from build123d import *

# Parameters (mm, degrees)
F0_R     = 1.905
F1_DEPTH = 5.08
F0_R_2   = 58.9915
F2_DEPTH = 10.16
F3_R     = 1.8415
F7_D     = 3.81
F7_DEPTH = 3.81
F7_TIP   = 1.1446394792


with BuildPart() as f1:
    # F0 (on Top) → F1 (new body)
    with BuildSketch(Plane.XY):
        Polygon((-6.4052528628, -3.7129219378), (-0.0261097385, -7.3959219378), (6.3530333858, -3.7129219378), (6.3530333858, 3.6530780622), (-0.0261097385, 7.3360780622), (-6.4052528628, 3.6530780622), align=None)
        with Locations((-0.0261097385, -0.0299219378)):
            Circle(F0_R, mode=Mode.SUBTRACT)
    extrude(amount=F1_DEPTH)

    # F0 (on Top) → F2 (join)
    with BuildSketch(Plane.XY):
        Circle(F0_R_2)
        with BuildLine():
            Line((-44.2124819173, 9.2097946363), (-23.9423226363, 4.6011586921))
            ThreePointArc((-23.9423226363, 4.6011586921), (-20.5137110236, 2.5239744907), (-19.0126005957, -1.1931129822))
            ThreePointArc((-19.0126005957, -1.1931129822), (-18.1042521178, -5.9277782732), (-16.0364137318, -10.2827979958))
            ThreePointArc((-16.0364137318, -10.2827979958), (-15.0448681501, -14.1162516757), (-16.5173341467, -17.7918976931))
            Line((-16.5173341467, -17.7918976931), (-29.9142206112, -33.7590248091))
            ThreePointArc((-29.9142206112, -33.7590248091), (-34.752324822, -36.0274693708), (-39.6091563625, -33.7994028387))
            ThreePointArc((-39.6091563625, -33.7994028387), (-49.423694035, -16.3885132924), (-51.9564452709, 3.4369601117))
            ThreePointArc((-51.9564452709, 3.4369601117), (-49.4154929179, 8.1088853878), (-44.2124819173, 9.2097946363))
        make_face(mode=Mode.SUBTRACT)
        Polygon((6.3530333858, -3.7129219378), (-0.0261097385, -7.3959219378), (-6.4052528628, -3.7129219378), (-6.4052528628, 3.6530780622), (-0.0261097385, 7.3360780622), (6.3530333858, 3.6530780622), align=None, mode=Mode.SUBTRACT)
        with BuildLine():
            ThreePointArc((-11.7881374723, -21.3045429378), (-8.7511162218, -18.7113231264), (-4.766540139, -18.4440395549))
            ThreePointArc((-4.766540139, -18.4440395549), (0, -19.05), (4.766540139, -18.4440395549))
            ThreePointArc((4.766540139, -18.4440395549), (8.7511162218, -18.7113231264), (11.7881374723, -21.3045429378))
            Line((11.7881374723, -21.3045429378), (22.5588981673, -39.1036858663))
            ThreePointArc((22.5588981673, -39.1036858663), (23.1511277222, -44.3967165208), (19.5047791508, -48.2788617334))
            ThreePointArc((19.5047791508, -48.2788617334), (0, -52.07), (-19.5047791508, -48.2788617334))
            ThreePointArc((-19.5047791508, -48.2788617334), (-23.1511277222, -44.3967165208), (-22.5588981673, -39.1036858663))
            Line((-22.5588981673, -39.1036858663), (-11.7881374723, -21.3045429378))
        make_face(mode=Mode.SUBTRACT)
        with Locations((53.3448168004, -15.4270773673)):
            Circle(F0_R, mode=Mode.SUBTRACT)
        with BuildLine():
            Line((29.9142206112, -33.7590248091), (16.5173341467, -17.7918976931))
            ThreePointArc((16.5173341467, -17.7918976931), (15.0448681501, -14.1162516757), (16.0364137318, -10.2827979958))
            ThreePointArc((16.0364137318, -10.2827979958), (18.1042521178, -5.9277782732), (19.0126005957, -1.1931129822))
            ThreePointArc((19.0126005957, -1.1931129822), (20.5137110236, 2.5239744907), (23.9423226363, 4.6011586921))
            Line((23.9423226363, 4.6011586921), (44.2124819173, 9.2097946363))
            ThreePointArc((44.2124819173, 9.2097946363), (49.4154929179, 8.1088853878), (51.9564452709, 3.4369601117))
            ThreePointArc((51.9564452709, 3.4369601117), (49.423694035, -16.3885132924), (39.6091563625, -33.7994028387))
            ThreePointArc((39.6091563625, -33.7994028387), (34.752324822, -36.0274693708), (29.9142206112, -33.7590248091))
        make_face(mode=Mode.SUBTRACT)
        with BuildLine():
            ThreePointArc((-12.3878761858, 50.5749485774), (-7.1524486585, 49.550133826), (-4.5459522271, 44.895445542))
            Line((-4.5459522271, 44.895445542), (-2.54, 18.8799073091))
            ThreePointArc((-2.54, 18.8799073091), (-9.267390723, 16.6438568003), (-14.7113573439, 12.1028288057))
            ThreePointArc((-14.7113573439, 12.1028288057), (-18.0767743108, 9.9762673559), (-22.0468294507, 10.2711523285))
            Line((-22.0468294507, 10.2711523285), (-41.2782743334, 18.243402288))
            ThreePointArc((-41.2782743334, 18.243402288), (-44.8916103761, 22.1650802153), (-44.2419474535, 27.4578765661))
            ThreePointArc((-44.2419474535, 27.4578765661), (-30.5832304695, 42.1420326284), (-12.3878761858, 50.5749485774))
        make_face(mode=Mode.SUBTRACT)
        with BuildLine():
            ThreePointArc((12.3878761858, 50.5749485774), (30.5832304695, 42.1420326284), (44.2419474535, 27.4578765661))
            ThreePointArc((44.2419474535, 27.4578765661), (44.8916103761, 22.1650802153), (41.2782743334, 18.243402288))
            Line((41.2782743334, 18.243402288), (22.0468294507, 10.2711523285))
            ThreePointArc((22.0468294507, 10.2711523285), (18.0767743108, 9.9762673559), (14.7113573439, 12.1028288057))
            ThreePointArc((14.7113573439, 12.1028288057), (9.267390723, 16.6438568003), (2.54, 18.8799073091))
            Line((2.54, 18.8799073091), (4.5459522271, 44.895445542))
            ThreePointArc((4.5459522271, 44.895445542), (7.1524486585, 49.550133826), (12.3878761858, 50.5749485774))
        make_face(mode=Mode.SUBTRACT)
        with Locations((53.3448168004, -15.4270773673)):
            Circle(F0_R)
    extrude(amount=F2_DEPTH)


with BuildPart() as f5:
    # F3 (on Front) → F5 (revolve)
    with BuildSketch(Plane.XZ):
        with Locations((59.055, 5.08)):
            Circle(F3_R)
    revolve(axis=Axis((0, 0, 4.4038342312), (0, 0, 1)))


with BuildPart() as f1_1:
    add(f1.part)

    # F6: cut F5
    add(f5.part, mode=Mode.SUBTRACT)

    # F7
    with Locations(Plane(origin=(0, 0, 0), x_dir=(1, 0, 0), z_dir=(0, 0, -1))):
        with Locations((53.3448168004, 15.4270773673)):
            Hole(F7_D / 2, depth=F7_DEPTH)
            with Locations((0, 0, -(F7_DEPTH + F7_TIP / 2))):  # 118° drill point
                Cone(0, F7_D / 2, F7_TIP, mode=Mode.SUBTRACT)


solid = f1_1.part
Model file for the job. Use its own axes, mm. A direction names the side the tool comes from. Coordinates: 2 decimals unless noted, no trailing zeros. Use one line per item in the form item = value. Start each with the question number.
(1) Tool access for faces 4 (the conical face through (53.273, -15.104, 4.756)), 5 (the flat face through (3.12, 5.52, 7.58)), 6 (the flat face through (-31.528, 14.201, 5.009)): list every direction of +Z, -Z, +X, -X, +Y, -Y with a clear straight run to the whole face (end or side of a thin tool).
(2) Probe probe 1 along Y at (x, z) = (-37, 9); probe 2 along X at (y, z) = (24, 4.25); probe 3 along Y at (x, z) = (-12, 1). List the from-to ranges inside material, lowest first. Write a range as from..to.
(3) Flat gauge pins, fed straight in: pin 1 (4 mm diameter, centred on x = 2.5, y = 0.5, fed in from +Z); pin 2 (6 mm diameter, centred on x = -45, z = 1.5, fed in from +Y); pin 3 (4 mm diameter, centred on x = -9.5, z = 7.5, fed in from +Y). Where does each tip first touch, or does it go through?
(4) Pull direction X, two halves, no side cores. Call faces 1 (the flat face through (12, 1, 0)), 2 (the cylindrical face through (-12.79, -57.59, 8.52)), 3 (the flat face through (3.53, 31.71, 5.01)): pulls with the +X half, pulls with the -X half, needs draft (parallel to the pull), parting line crosses it, or undercut.
(5) Cut at A-A on y = 30.5. Give the number of separate pieces and of enclosed holes in the cut face, and give its area (3 significant figures).
Values:
q1.face_4 = -Z
q1.face_5 = +Z
q1.face_6 = +Z, -Z
q2.probe_1 = -45.95..-35.63, 7.57..16.47, 36.64..45.95
q2.probe_2 = -52.15..-45.2, -2.93..2.93, 45.2..52.15
q2.probe_3 = -57.76..-50.67, -21.65..14.8, 50.66..57.76
q3.pin_1 = 5.08
q3.pin_2 = 41.42
q3.pin_3 = 58.51
q4.face_1 = needs draft
q4.face_2 = parting line crosses it
q4.face_3 = undercut
q5.separate_pieces = 3
q5.enclosed_holes = 0
q5.area = 226 mm2
